```python
from build123d import *

# Parameters (mm, degrees)
SHS_C450_AS_50X50X2_3_SHS_C450_1_DEPTH = 800
CUT_EXTRUDE1_DEPTH                     = 402.559460105
CUT_EXTRUDE1_DEPTH_BACK                = 402.559460105
SKETCH20_W                             = 45
SKETCH20_H                             = 45
SKETCH21_R                             = 3.25
CUT_EXTRUDE2_DEPTH                     = 10
SKETCH22_R                             = 3.25
CUT_EXTRUDE3_DEPTH                     = 404.887360535
SKETCH23_R                             = 3.25
CUT_EXTRUDE4_DEPTH                     = 404.887360535


with BuildPart() as part:
    # Sketch19 → Shs c450 as 50X50X2.3 SHS C450(1) (new body)
    with BuildSketch(Plane.YZ.offset(-400)):
        with BuildLine():
            Line((-20.4, -25), (20.4, -25))
            ThreePointArc((20.4, -25), (23.652691193, -23.652691193), (25, -20.4))
            Line((25, -20.4), (25, 20.4))
            ThreePointArc((25, 20.4), (23.652691193, 23.652691193), (20.4, 25))
            Line((20.4, 25), (-20.4, 25))
            ThreePointArc((-20.4, 25), (-23.652691193, 23.652691193), (-25, 20.4))
            Line((-25, 20.4), (-25, -20.4))
            ThreePointArc((-25, -20.4), (-23.652691193, -23.652691193), (-20.4, -25))
        make_face()
        with BuildLine():
            Line((-20.4, 22.7), (20.4, 22.7))
            ThreePointArc((20.4, 22.7), (22.026345597, 22.026345597), (22.7, 20.4))
            Line((22.7, 20.4), (22.7, -20.4))
            ThreePointArc((22.7, -20.4), (22.026345597, -22.026345597), (20.4, -22.7))
            Line((20.4, -22.7), (-20.4, -22.7))
            ThreePointArc((-20.4, -22.7), (-22.026345597, -22.026345597), (-22.7, -20.4))
            Line((-22.7, -20.4), (-22.7, 20.4))
            ThreePointArc((-22.7, 20.4), (-22.026345597, 22.026345597), (-20.4, 22.7))
        make_face(mode=Mode.SUBTRACT)
    extrude(amount=SHS_C450_AS_50X50X2_3_SHS_C450_1_DEPTH)

    # Sketch20 → Cut-Extrude1 (cut, two sides: drawn at the far end of the back side and taken through both)
    with BuildSketch(Plane(origin=(0, 0, 0), x_dir=(1, 0, 0), z_dir=(0, 1, 0)).offset(-CUT_EXTRUDE1_DEPTH_BACK)):
        with Locations((-377.5, -2.5)):
            Rectangle(SKETCH20_W, SKETCH20_H)
        with Locations((377.5, -2.5)):
            Rectangle(SKETCH20_W, SKETCH20_H)
    extrude(amount=CUT_EXTRUDE1_DEPTH + CUT_EXTRUDE1_DEPTH_BACK, mode=Mode.SUBTRACT)

    # Sketch21 → Cut-Extrude2 (cut)
    with BuildSketch(Plane(origin=(0, 0, -25), x_dir=(-1, 0, 0), z_dir=(0, 0, -1))):
        with Locations((-375, 0)):
            Circle(SKETCH21_R)
        with Locations((375, 0)):
            Circle(SKETCH21_R)
    extrude(amount=-CUT_EXTRUDE2_DEPTH, mode=Mode.SUBTRACT)

    # Sketch22 → Cut-Extrude3 (cut, through all)
    with BuildSketch(Plane.XY.offset(25)):
        with Locations((-155.7, 0)):
            Circle(SKETCH22_R)
        with Locations((-100.7, 0)):
            Circle(SKETCH22_R)
    extrude(amount=-CUT_EXTRUDE3_DEPTH, mode=Mode.SUBTRACT)

    # Sketch23 → Cut-Extrude4 (cut, through all)
    with BuildSketch(Plane(origin=(0, 25, 0), x_dir=(1, 0, 0), z_dir=(0, 1, 0))):
        with Locations(Location((-203.2, 0, 0), (0, 0, 180))):
            Circle(SKETCH23_R)
        with Locations(Location((-53.2, 0, 0), (0, 0, 180))):
            Circle(SKETCH23_R)
    extrude(amount=-CUT_EXTRUDE4_DEPTH, mode=Mode.SUBTRACT)


solid = part.part
```
Work out the finished part from the listing and answer in its coordinate system (mm). A direction names the side the tool comes from. Round coordinates to 2 decimals unless told otherwise and drop trailing zeros. Write each loop counter-clockwise with the first axis right and the second up, starting at its lowest first coordinate (ties: lowest second). Pieces come first, ordered by that corner, then holes. Notation, with made-up numbers: (42, 0) -> (100, 0) arc R20 cw to (100, 21) -> close; hole circle Ø1 at (28, 9). An arc over 180 degrees is marked (long way). Write each question's results on one line, items separated by ' | '.
Q1. Which of the six approach directions +Z, -Z, +X, -X, +Y, -Y give full straight-line access (tool end or side, diameter ignored) to faces 5 (the flat face through (-6, 0, -25)), 6 (the flat face through (355, 0, 24)), 7 (the flat face through (-6, 25, 0)), 8 (the flat face through (-6, 0, -22.7)), 9 (the flat face through (-355, 0, 24))?
Data:
face 5: -Z, +X, -X, +Y, -Y | face 6: +Z, +X, +Y, -Y | face 7: +Z, -Z, +X, -X, +Y | face 8: +X, -X | face 9: +Z, -X, +Y, -Y
Q2. Determine the mould class of faces 1 (the flat face through (-5, 0, 25)), 2 (the flat face through (-6, -22.7, 0)), 3 (the flat face through (-6, -25, 0)), 4 (the flat face through (-5, 0, 22.7)) for opening direction Y: released by +Y, released by -Y, zero draft, split by the parting line, or undercut.
Data:
face 1: zero draft | face 2: undercut | face 3: released by -Y | face 4: undercut
Q3. Flat-ended cylindrical pins translate along their axes: P1, Ø1.8, axis at x = -369, y = -23.5, coming from the +Z side; P2, Ø12, axis at y = -2, z = 19, coming from the +X side; P3, Ø12, axis at y = 17, z = 15.5, coming from the -X side. Find the tip coordinate at first contact, or state that the pin passes through.
Data:
P1: z = -20 | P2: x = 355 | P3: x = -355
Q4. Straight lines are drawn through the part: line 1 along Z through (x, y) = (-63.5, -2.5); line 2 along Z through (x, y) = (-203, 23). For each, find the intervals that lie inside material, in ascending order. Write a range as [from, to].
Data:
line 1: [-25, -22.7], [22.7, 25] | line 2: [-24.19, -3.24], [3.24, 24.19]
Q5. Section A-A, the plane x = 124 is taken. Write down the section's boundary in (y, z), then the cut area to 3 significant figures.
Data:
outline: (-25, -20.4) arc R4.6 ccw to (-20.4, -25) -> (20.4, -25) arc R4.6 ccw to (25, -20.4) -> (25, 20.4) arc R4.6 ccw to (20.4, 25) -> (-20.4, 25) arc R4.6 ccw to (-25, 20.4) -> close; hole (-22.7, -20.4) arc R2.3 ccw to (-20.4, -22.7) -> (20.4, -22.7) arc R2.3 ccw to (22.7, -20.4) -> (22.7, 20.4) arc R2.3 ccw to (20.4, 22.7) -> (-20.4, 22.7) arc R2.3 ccw to (-22.7, 20.4) -> close | area: 425 mm^2
